Geometry: see drawing. Coordinates: mm, zero at the bounding-box minimum. Coordinates: 2 decimals unless noted, no trailing zeros. Write each loop counter-clockwise with the first axis right and the second up, starting at its lowest first coordinate (ties: lowest second). Pieces come first, ordered by that corner, then holes. Notation, with made-up numbers: (-19.5, -12) - (-8.5, -12) arc R25 ccw to (-8.5, 9) - close; hole circle Ø7 at (39, 84.5). An arc over 180 degrees is marked (long way). One line per question, with ' | ' between items. Start each with the question number.
Q1. Cut plane B-B, the plane x = 77. Return loops of the section in (y, z) (1 decimal), plus the area to 3 significant figures.
Q2. Cut plane A-A, the plane y = 4. Give the number of separate pieces and of enclosed holes in the cut face, plus the area to 3 significant figures.
Q3. Cut plane C-C, the plane z = 161.5. Return loops of the section in (x, y), plus the area to 3 significant figures.
Q4. Contact query for flat-ended pins moving along their axis: P1, Ø1.5, axis at y = 12, z = 368, coming from the -X side; P2, Ø12, axis at x = 437, z = 172.5, coming from the -Y side; P3, Ø5, axis at x = 442.69, z = 361.25, coming from the +Y side; P4, Ø10, axis at y = 13, z = 290, coming from the -X side. Output: stop coordinate, or through.
Q5. Line query: line 1 (X direction, y = 4, z = 250); line 2 (Z direction, x = 57.5, y = 14) (1 decimal). Output: solid intervals per line, ascending.
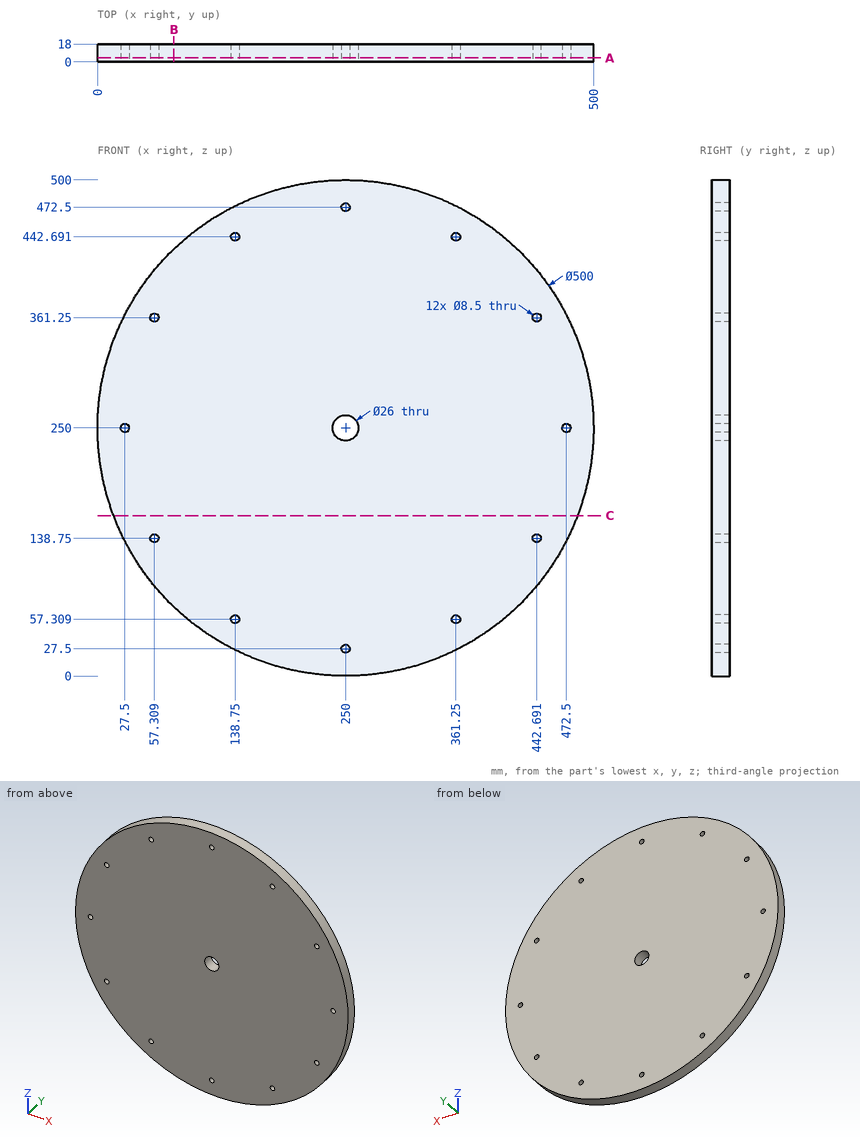
Reply:
1) outline: (0, 69.5) - (18, 69.5) - (18, 430.5) - (0, 430.5) - close | area: 6,500 mm^2
2) separate pieces: 1 | enclosed holes: 13 | area: 195,000 mm^2
3) outline: (16.19, 0) - (483.81, 0) - (483.81, 18) - (16.19, 18) - close | area: 8,420 mm^2
4) P1: stops at x = 29.2 | P2: stops at y = 0 | P3: passes through | P4: stops at x = 2.46
5) line 1: x = 0 to 23.25, 31.75 to 237, 263 to 468.25, 476.75 to 500 | line 2: z = 90.5 to 134.5, 143 to 357, 365.5 to 409.5
